```python
from build123d import *

# Parameters (mm, degrees)
SKETCH2_W           = 120
SKETCH2_H           = 120
BOSS_EXTRUDE1_DEPTH = 30
SKETCH4_R           = 35
BOSS_EXTRUDE2_DEPTH = 25
SKETCH6_R           = 25
CUT_EXTRUDE1_DEPTH  = 179.395627749
FILLET1_R           = 5
FILLET2_R           = 1.5


with BuildPart() as part:
    # Sketch2 → Boss-Extrude1 (new body)
    with BuildSketch(Plane.XY):
        with Locations((60, 60)):
            Rectangle(SKETCH2_W, SKETCH2_H)
    extrude(amount=BOSS_EXTRUDE1_DEPTH)

    # Sketch4 → Boss-Extrude2 (add)
    with BuildSketch(Plane.XY.offset(30)):
        with Locations(Location((60, 60, 0), (0, 0, 180))):
            Circle(SKETCH4_R)
    extrude(amount=BOSS_EXTRUDE2_DEPTH)

    # Sketch6 → Cut-Extrude1 (cut, through all)
    with BuildSketch(Plane.XY.offset(55)):
        with Locations((60, 60)):
            Circle(SKETCH6_R)
    extrude(amount=-CUT_EXTRUDE1_DEPTH, mode=Mode.SUBTRACT)

    # Fillet1
    fillet1_edges = [part.edges().sort_by_distance(p)[0] for p in [
        (120, 60, 30),
        (60, 120, 30),
        (95, 60, 30),
        (0, 60, 30),
        (60, 0, 30),
        (0, 120, 15),
        (120, 120, 15),
        (120, 0, 15),
        (0, 0, 15),
    ]]
    fillet(fillet1_edges, radius=FILLET1_R)

    # Fillet2
    fillet2_edges = [part.edges().sort_by_distance(p)[0] for p in [
        (95, 60, 55),
        (35, 60, 55),
    ]]
    fillet(fillet2_edges, radius=FILLET2_R)


solid = part.part
```
The model under review builds one solid part; all positions refer to its coordinate system, in mm. A direction names the side the tool comes from. Coordinates: 2 decimals unless noted, no trailing zeros. Order: outer loops, then holes, each group sorted by start corner. A loop starts at its lowest first (then second) coordinate and runs counter-clockwise, first axis right, second up. Notation, with made-up numbers: (75.5, 28) -> (133.5, 28) arc R38 cw to (133.5, 66) -> close; hole circle Ø9 at (41, 75). An arc over 180 degrees is marked (long way). Answer in a Markdown table with one row per item. Add a question column.
Item 1: We need section A-A on z = 28. Write out the cut boundary in (x, y).
Item 2: We need section D-D on x = 14. Write out the cut boundary in (y, z), plus the area to 3 significant figures.
Item 3: We need section B-B on x = 60. Write out the cut boundary in (y, z), plus the area to 3 significant figures.
Item 4: Clearance check with flat-ended pins moving along their axes: pin 1 (1.5 mm diameter, centred on x = 65.5, z = 35, fed in from -Y); pin 2 (6 mm diameter, centred on y = 95.5, z = 32, fed in from +X). State where each tip first meets the part, or that it passes through.
Item 5: Mouldability with a two-part tool opening along Y and no side actions: class faces 1 (the cylindrical face through (41.574, 76.896, 27.124)), 2 (the cylindrical face through (1, 61, 28)), 3 (the cylindrical face through (118, 119, 13)) as +Y half, -Y half, draft (parallel to the pull), parting line (faces both ways), or undercut.
Item 6: Machinability: for faces 4 (the flat face through (35, 97, 30)), 5 (the flat face through (0, 59, 12)), which of the approach directions +Z, -Z, +X, -X, +Y, -Y give a long, thin tool a straight path to every point of the face, cutting with its end or side? Answer none if there is none.
Item 7: To check wall thickness, follow probe 1 along Y at (x, z) = (60, 41); probe 2 along Z at (x, y) = (31, 96.5); probe 3 along Y at (x, z) = (60, 18). State the ranges of each line that lie inside material, in increasing order.
Final values:
| question | item | result |
|---|---|---|
| 1 | outline | (1, 5) arc R4 ccw to (5, 1) -> (115, 1) arc R4 ccw to (119, 5) -> (119, 115) arc R4 ccw to (115, 119) -> (5, 119) arc R4 ccw to (1, 115) -> close; hole circle Ø50 at (60, 60) |
| 2 | outline | (0, 0) -> (120, 0) -> (120, 25) arc R5 ccw to (115, 30) -> (5, 30) arc R5 ccw to (0, 25) -> close |
| 2 | area | 3,590 mm2 |
| 3 | outline | (0, 0) -> (35, 0) -> (35, 53.5) arc R1.5 ccw to (33.5, 55) -> (26.5, 55) arc R1.5 ccw to (25, 53.5) -> (25, 35) arc R5 cw to (20, 30) -> (5, 30) arc R5 ccw to (0, 25) -> close; (85, 0) -> (120, 0) -> (120, 25) arc R5 ccw to (115, 30) -> (100, 30) arc R5 cw to (95, 35) -> (95, 53.5) arc R1.5 ccw to (93.5, 55) -> (86.5, 55) arc R1.5 ccw to (85, 53.5) -> close |
| 3 | area | 2,600 mm2 |
| 4 | pin 1 | stops at y = 25.32 |
| 4 | pin 2 | stops at x = 118 |
| 5 | face 1 | undercut |
| 5 | face 2 | draft |
| 5 | face 3 | +Y half |
| 6 | face 4 | +Z |
| 6 | face 5 | +Z, -Z, -X, +Y, -Y |
| 7 | probe 1 | y = 25 to 35, 85 to 95 |
| 7 | probe 2 | z = 0 to 30 |
| 7 | probe 3 | y = 0 to 35, 85 to 120 |
